For this review, take the finished solid that the model builds, in its own axes (mm). A direction names the side the tool comes from. Round coordinates to 2 decimals unless told otherwise and drop trailing zeros. Order: outer loops, then holes, each group sorted by start corner. A loop starts at its lowest first (then second) coordinate and runs counter-clockwise, first axis right, second up. Notation, with made-up numbers: (61.25, 85) -> (67.25, 85) arc R27 ccw to (67.25, 124) -> close; hole circle Ø11 at (44, 50.5). An arc over 180 degrees is marked (long way). Answer in a Markdown table with one row per item.
```python
from build123d import *

# Parameters (mm, degrees)
BASEHEAD_DEPTH = 12.5


with BuildPart() as part:
    # Sketch1 → BaseHead (new body)
    with BuildSketch(Plane(origin=(0, 0, 0), x_dir=(0, 0, -1), z_dir=(1, 0, 0))):
        Polygon((15, 8.660254038), (15, -8.660254038), (0, -17.320508076), (-15, -8.660254038), (-15, 8.660254038), (0, 17.320508076), align=None)
    extrude(amount=BASEHEAD_DEPTH)

    # BodySke → BaseBody (revolve)
    with BuildSketch(Plane.XY):
        Polygon((0, 0), (102.5, 0), (102.5, 8.626), (101.126, 10), (0, 10), align=None)
    revolve(axis=Axis((0, 0, 0), (1, 0, 0)))

    # Sketch3 → HeadChamfer (revolve, cut)
    with BuildSketch(Plane.XY):
        Polygon((0, 15), (4.226497308, 22.320508076), (4.226497308, 27.320508076), (-10, 27.320508076), (-10, 15), align=None)
    revolve(axis=Axis((0, 0, 0), (1, 0, 0)), mode=Mode.SUBTRACT)


solid = part.part
```
Q1. Take a section at A-A, the plane x = 37.5. Write out the cut boundary in (y, z).
Answer key:
| item | result |
|---|---|
| outline | circle Ø20 at (0, 0) |
Q2. Clearance check with flat-ended pins moving along their axes: pin 1 Ø1 at (x, y) = (55, -7.5) entering from -Z; pin 2 Ø1.5 at (x, z) = (28, 1) entering from +Y; pin 3 Ø6 at (x, y) = (74, -2) entering from -Z; pin 4 Ø12 at (y, z) = (-14, -3.5) entering from -X. State where each tip first meets the part, or that it passes through.
Answer key:
| item | result |
|---|---|
| pin 1 | stops at z = -7.14 |
| pin 2 | stops at y = 10 |
| pin 3 | stops at z = -10 |
| pin 4 | stops at x = 0 |
Q3. To check wall thickness, follow probe 1 along X at (y, z) = (-8.5, -10); probe 2 along Z at (x, y) = (60, -2.5); probe 3 along X at (y, z) = (8, 3.25). State the ranges of each line that lie inside material, in increasing order.
Answer key:
| item | result |
|---|---|
| probe 1 | x = 0 to 12.5 |
| probe 2 | z = -9.68 to 9.68 |
| probe 3 | x = 0 to 102.49 |
Q4. Tool access review of faces 1 (the face through (6.163, 12.93, 7.605)), 2 (the face through (12.5, -7.5, -6.9)): name each direction out of +Z, -Z, +X, -X, +Y, -Y from which nothing blocks a thin tool from reaching the whole face with its end or side.
Answer key:
| item | result |
|---|---|
| face 1 | +Z, +X, -X, +Y |
| face 2 | +X |
